Work out the finished part from the listing and answer in its coordinate system (mm). A direction names the side the tool comes from. Round coordinates to 2 decimals unless told otherwise and drop trailing zeros. Loops run counter-clockwise (first coordinate to the right, second up) from the corner with the lowest first, then second, coordinate; pieces in that order, holes last. Notation, with made-up numbers: (72.5, 49) -> (130.5, 49) arc R13 ccw to (130.5, 67) -> close; hole circle Ø11 at (25, 32). An arc over 180 degrees is marked (long way). Use CSV: the item, a comma, the result in double quotes. Start each with the question number.
from build123d import *

# Parameters (mm, degrees)
F1_DEPTH       = 12
F2_D           = 5.5
F2_CBORE_D     = 9.75
F2_CBORE_DEPTH = 5
F3_R           = 4.99999


# Not quite as in the source:
# - a fillet or chamfer is up to 0.001 mm smaller than in the source, because OpenCascade refuses the exact size


with BuildPart() as f1:
    # F0 (on Top) → F1 (new body)
    with BuildSketch(Plane.XY):
        with BuildLine():
            Line((84.472135955, 8.94427191), (4.472135955, 48.94427191))
            ThreePointArc((4.472135955, 48.94427191), (-5.2573111212, 48.5065080835), (-10, 40))
            Line((-10, 40), (-10, -40))
            ThreePointArc((-10, -40), (-5.2573111212, -48.5065080835), (4.472135955, -48.94427191))
            Line((4.472135955, -48.94427191), (84.472135955, -8.94427191))
            ThreePointArc((84.472135955, -8.94427191), (90, 0), (84.472135955, 8.94427191))
        make_face()
        with BuildLine():
            Line((10, -31.7639320225), (10, -12))
            ThreePointArc((10, -12), (10.5857864376, -10.5857864376), (12, -10))
            Line((12, -10), (51.527864045, -10))
            ThreePointArc((51.527864045, -10), (53.4743620239, -11.5404941589), (52.422291236, -13.788854382))
            Line((52.422291236, -13.788854382), (12.894427191, -33.5527864045))
            ThreePointArc((12.894427191, -33.5527864045), (10.9485377758, -33.4652336392), (10, -31.7639320225))
        make_face(mode=Mode.SUBTRACT)
        with BuildLine():
            ThreePointArc((10, 31.7639320225), (10.9485377758, 33.4652336392), (12.894427191, 33.5527864045))
            Line((12.894427191, 33.5527864045), (52.422291236, 13.788854382))
            ThreePointArc((52.422291236, 13.788854382), (53.4743620239, 11.5404941589), (51.527864045, 10))
            Line((51.527864045, 10), (12, 10))
            ThreePointArc((12, 10), (10.5857864376, 10.5857864376), (10, 12))
            Line((10, 12), (10, 31.7639320225))
        make_face(mode=Mode.SUBTRACT)
    extrude(amount=F1_DEPTH)

    # F2 (through all)
    with Locations(Plane(origin=(0, 0, 0), x_dir=(1, 0, 0), z_dir=(0, 0, -1))):
        with Locations((0, -40), (0, 40), (0, 0), (40, 0), (80, 0)):
            CounterBoreHole(F2_D / 2, F2_CBORE_D / 2, F2_CBORE_DEPTH)

    # F3 (radius 5 in the source; OpenCascade refuses exactly that, so slightly less here)
    f3_edges = [f1.edges().sort_by_distance(p)[0] for p in [
        (44.472136, 28.944272, 0),
        (32.658359, 23.67082, 0),
        (32.658359, -23.67082, 0),
    ]]
    fillet(f3_edges, radius=F3_R)


solid = f1.part
Q1. Straight lines are drawn through the part: line 1 (Y direction, x = 0, z = 7); line 2 (Y direction, x = 0, z = 2.85) (3 decimals); line 3 (Y direction, x = 52.5, z = 11.25). For each, find the intervals that lie inside material, in ascending order. Write a range as from..to.
Q2. Section B-B, the plane z = 7 is taken. Write down the section's boundary in (x, y).
Q3. For a pull along X with two mould halves and no side action, classify faces 1 (the flat face through (2.1, 42.1, 5)), 2 (the cylindrical face through (44.39, -27.39, 1.5)), 3 (the flat face through (-10, 1, 8)) as pulls with the +X half, pulls with the -X half, needs draft (parallel to the pull), parting line crosses it, or undercut.
Q4. Each of these flat-tipped pins is pushed along its axis until it touches: pin 1 (11 mm diameter, centred on x = 0, y = 0, fed in from +Z); pin 2 (5.5 mm diameter, centred on y = -18, z = 9.5, fed in from +X); pin 3 (3.5 mm diameter, centred on x = 35, z = 8.5, fed in from -Y); pin 4 (2 mm diameter, centred on y = 7.5, z = 6.5, fed in from +X). Where does it stop, or does it pass through?
Q5. Section D-D, the plane z = 1.75 is taken. Write down the section's boundary in (x, y) (3 decimals).
Q6. Section A-A, the plane y = 0 is taken. Give the number of separate pieces and of enclosed holes in the cut face, and give its area (3 significant figures).
Q7. Which of the six approach directions +Z, -Z, +X, -X, +Y, -Y give full straight-line access (tool end or side, diameter ignored) to faces 4 (the flat face through (32, 10, 8)), 5 (the cylindrical face through (90, 0, 8)), 6 (the flat face through (42.1, 2.1, 5))?
Report:
1,line 1,"y = -50..-42.75, -37.25..-2.75, 2.75..37.25, 42.75..50"
1,line 2,"y = -49.514..-44.875, -35.125..-4.875, 4.875..35.125, 44.875..49.514"
1,line 3,"y = -24.93..-13.75, -10.25..10.25, 13.75..24.93"
2,outline,"(-10, -40) arc R10 ccw to (4.47, -48.94) -> (84.47, -8.94) arc R10 ccw to (84.47, 8.94) -> (4.47, 48.94) arc R10 ccw to (-10, 40) -> close; hole circle Ø5.5 at (0, -40); hole circle Ø5.5 at (0, 0); hole circle Ø5.5 at (0, 40); hole (10, -31.76) arc R2 ccw to (12.89, -33.55) -> (52.42, -13.79) arc R2 ccw to (51.53, -10) -> (12, -10) arc R2 ccw to (10, -12) -> close; hole (10, 12) arc R2 ccw to (12, 10) -> (51.53, 10) arc R2 ccw to (52.42, 13.79) -> (12.89, 33.55) arc R2 ccw to (10, 31.76) -> close; hole circle Ø5.5 at (40, 0); hole circle Ø5.5 at (80, 0)"
3,face 1,"undercut"
3,face 2,"pulls with the +X half"
3,face 3,"pulls with the -X half"
4,pin 1,"stops at z = 12"
4,pin 2,"stops at x = 71.86"
4,pin 3,"stops at y = -34.56"
4,pin 4,"stops at x = 87.6"
5,outline,"(-8.8, -40) arc R8.8 ccw to (3.935, -47.871) -> (83.935, -7.871) arc R8.8 ccw to (83.935, 7.871) -> (3.935, 47.871) arc R8.8 ccw to (-8.8, 40) -> close; hole circle Ø9.75 at (0, -40); hole circle Ø9.75 at (0, 0); hole circle Ø9.75 at (0, 40); hole (8.8, -31.764) arc R3.2 ccw to (13.431, -34.626) -> (52.959, -14.862) arc R3.2 ccw to (51.528, -8.8) -> (12, -8.8) arc R3.2 ccw to (8.8, -12) -> close; hole (8.8, 12) arc R3.2 ccw to (12, 8.8) -> (51.528, 8.8) arc R3.2 ccw to (52.959, 14.862) -> (13.431, 34.626) arc R3.2 ccw to (8.8, 31.764) -> close; hole circle Ø9.75 at (40, 0); hole circle Ø9.75 at (80, 0)"
6,separate pieces,"4"
6,enclosed holes,"0"
6,area,"928 mm²"
7,face 4,"+Z, -Z"
7,face 5,"+Z, -Z, +X"
7,face 6,"-Z"
